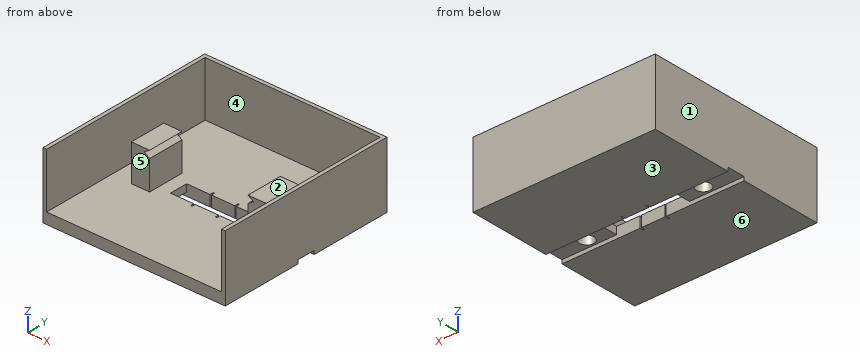
from build123d import *

# Parameters (mm, degrees)
SKICA1_W                 = 50
SKICA1_H                 = 50
P_IDAT_VYSUNUT_M2_DEPTH  = 3
SKICA4_W                 = 20
SKICA4_H                 = 5
ODEBRAT_VYSUNUT_M1_DEPTH = 2
SKICA5_W                 = 50
SKICA5_H                 = 5
ODEBRAT_VYSUNUT_M3_DEPTH = 1
SKICA10_W                = 5
SKICA10_H                = 10
P_IDAT_VYSUNUT_M6_DEPTH  = 10
ODEBRAT_VYSUNUT_M6_DEPTH = 10
P_IDAT_VYSUNUT_M9_DEPTH  = 15
SKICA16_W                = 0.4
SKICA16_H                = 7
ODEBRAT_VYSUNUT_M7_DEPTH = 10
SKICA17_R                = 2
ODEBRAT_VYSUNUT_M8_DEPTH = 4


with BuildPart() as part:
    # Skica1 → Přidat vysunutím2 (new body)
    with BuildSketch(Plane.XY):
        Rectangle(SKICA1_W, SKICA1_H)
    extrude(amount=P_IDAT_VYSUNUT_M2_DEPTH)

    # Skica4 → Odebrat vysunutím1 (cut)
    with BuildSketch(Plane.XY.offset(3)):
        Rectangle(SKICA4_W, SKICA4_H)
    extrude(amount=-ODEBRAT_VYSUNUT_M1_DEPTH, mode=Mode.SUBTRACT)

    # Skica5 → Odebrat vysunutím3 (cut)
    with BuildSketch(Plane(origin=(0, 0, 0), x_dir=(-1, 0, 0), z_dir=(0, 0, -1))):
        Rectangle(SKICA5_W, SKICA5_H)
    extrude(amount=-ODEBRAT_VYSUNUT_M3_DEPTH, mode=Mode.SUBTRACT)

    # Skica10 → Přidat vysunutím6 (add)
    with BuildSketch(Plane.XY.offset(3)):
        with Locations((-16, 0)):
            Rectangle(SKICA10_W, SKICA10_H)
        with Locations((16, 0)):
            Rectangle(SKICA10_W, SKICA10_H)
    extrude(amount=P_IDAT_VYSUNUT_M6_DEPTH)

    # Skica12 → Odebrat vysunutím6 (cut)
    with BuildSketch(Plane(origin=(0, 5, 0), x_dir=(1, 0, 0), z_dir=(0, 1, 0))):
        Polygon((-13.5, -13), (-13.5, -11), (-15, -12), align=None)
        Polygon((13.5, -13), (13.5, -11), (15, -12), align=None)
    extrude(amount=-ODEBRAT_VYSUNUT_M6_DEPTH, mode=Mode.SUBTRACT)

    # Skica14 → Přidat vysunutím9 (add)
    with BuildSketch(Plane.XY.offset(3)):
        Polygon((25, 25), (-25, 25), (-25, -25), (-24, -25), (-24, 24), (24, 24), (24, -25), (25, -25), align=None)
    extrude(amount=P_IDAT_VYSUNUT_M9_DEPTH)

    # Skica16 → Odebrat vysunutím7 (cut)
    with BuildSketch(Plane(origin=(0, 0, 0), x_dir=(-1, 0, 0), z_dir=(0, 0, -1))):
        with Locations((-3.4, 0)):
            Rectangle(SKICA16_W, SKICA16_H)
        with Locations((3.4, 0)):
            Rectangle(SKICA16_W, SKICA16_H)
    extrude(amount=-ODEBRAT_VYSUNUT_M7_DEPTH, mode=Mode.SUBTRACT)

    # Skica17 → Odebrat vysunutím8 (cut)
    with BuildSketch(Plane(origin=(0, 0, 1), x_dir=(-1, 0, 0), z_dir=(0, 0, -1))):
        with Locations((-16, 0)):
            Circle(SKICA17_R)
        with Locations((16, 0)):
            Circle(SKICA17_R)
    extrude(amount=-ODEBRAT_VYSUNUT_M8_DEPTH, mode=Mode.SUBTRACT)


solid = part.part
Design review of the part built by this model. Coordinates are the model's own, in mm. Face numbers are marked on the shaded views. A direction names the side the tool comes from. Give positions to 0.01 mm unless a question says otherwise; leave off trailing zeros. Loops run counter-clockwise (first coordinate to the right, second up) from the corner with the lowest first, then second, coordinate; pieces in that order, holes last. Notation, with made-up numbers: M 74,36.25 L 114,36.25 A5 ccw 114,45.25 Z; hole C -12.75,0 d5. An arc over 180 degrees is marked long. One line per question, with ' | ' between items. Start each with the question number.
1. To check wall thickness, follow L1, parallel to X at y = -21.5, z = 6.75; L2, parallel to Y at x = 16, z = 2.4; L3, parallel to Y at x = 15.5, z = 14.5. State the ranges of each line that lie inside material, in increasing order.
2. Add section D-D (z = 16). Write out the cut boundary in (x, y), plus the area to 3 significant figures.
3. The part is to be moulded in two halves that separate along X. For the marked faces 1, 2 and 3, say which applies: released by +X, released by -X, zero draft, split by the parting line, or undercut.
4. Insertion check: P1, Ø6, axis at x = -15.5, z = 9, coming from the -Y side; P2, Ø5.5, axis at x = 14.5, y = -1, coming from the -Z side; P3, Ø2, axis at x = 12, y = -11.5, coming from the +Z side. Each pin has a flat end and moves straight along its axis. Give the tip position at first contact, or say it passes through.
5. For the marked faces 4, 5 and 6, list the 3-axis set-ups (+Z, -Z, +X, -X, +Y, -Y) from which the entire face can be reached by the end or side of a thin tool; tool diameter is ignored.
6. Add section C-C (x = -12). Write out the cut boundary in (y, z).
7. Add section B-B (x = 7). Write out the cut boundary in (y, z), plus the area to 3 significant figures.
Worked out:
1) L1: x = -25 to -24, 24 to 25 | L2: y = -25 to -2, 2 to 25 | L3: y = 24 to 25
2) outline: M -25,-25 L -24,-25 L -24,24 L 24,24 L 24,-25 L 25,-25 L 25,25 L -25,25 Z | area: 148 mm²
3) face 1: released by -X | face 2: undercut | face 3: zero draft
4) P1: stops at y = -5 | P2: stops at z = 0 | P3: stops at z = 3
5) face 4: +Z | face 5: +Z, -Y | face 6: -Z, +X, -X, +Y, -Y
6) outline: M -25,0 L -2.5,0 L -2.5,1 L 2.5,1 L 2.5,0 L 25,0 L 25,18 L 24,18 L 24,3 L -25,3 Z
7) outline: M -25,0 L -2.5,0 L -2.5,3 L -25,3 Z; M 2.5,0 L 25,0 L 25,18 L 24,18 L 24,3 L 2.5,3 Z | area: 150 mm²
